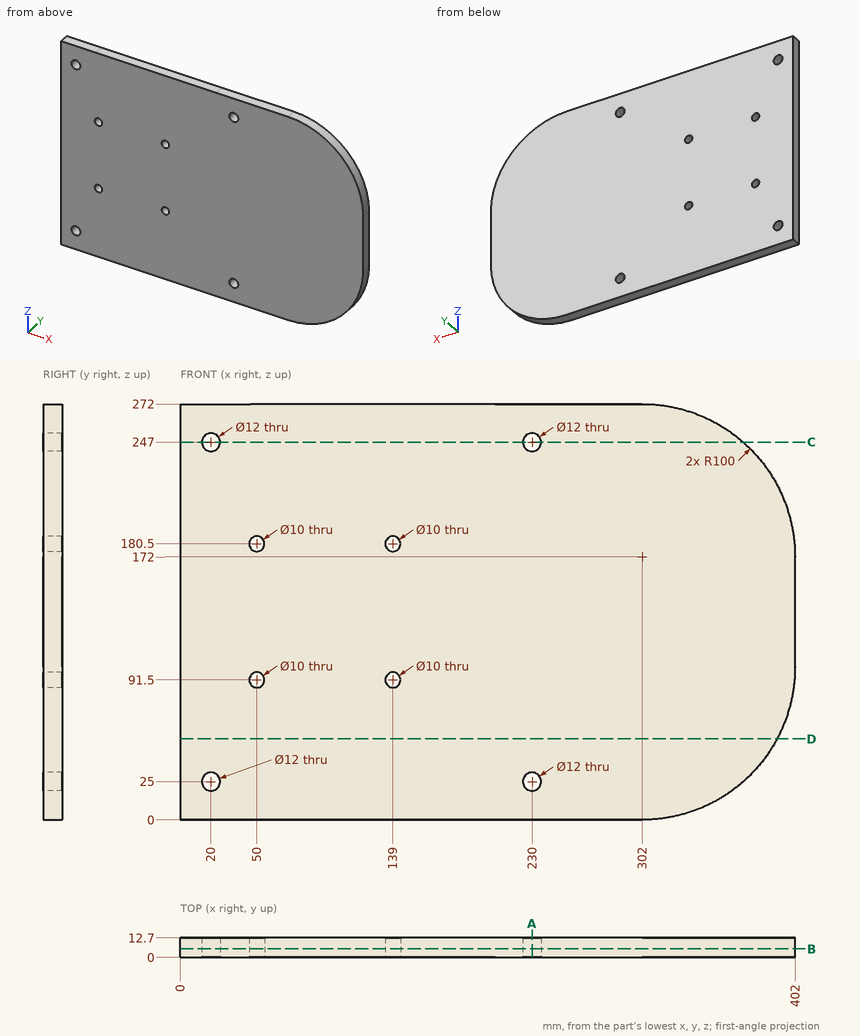
Geometry check sheet. Reference: drawing and pictorial views, mm from the part's lowest x, y, z. Round coordinates to 2 decimals unless told otherwise and drop trailing zeros. Order: outer loops, then holes, each group sorted by start corner. A loop starts at its lowest first (then second) coordinate and runs counter-clockwise, first axis right, second up. Notation, with made-up numbers: M 33,-28 L 44,-28 A30 cw 44,-2 Z; hole C -23,-32 d6. An arc over 180 degrees is marked long. Answer in a Markdown table with one row per item.
(1) Scan lines: probe 1 along Z at (x, y) = (50, 6.75); probe 2 along Z at (x, y) = (20, 9.75); probe 3 along X at (y, z) = (9.75, 180.5). Record each from-to range of solid material in increasing order. Write a range as from..to.
Responses:
| item | result |
|---|---|
| probe 1 | z = 0..86.5, 96.5..175.5, 185.5..272 |
| probe 2 | z = 0..19, 31..241, 253..272 |
| probe 3 | x = 0..45, 55..134, 144..401.64 |
(2) Sectioned sample at B-B, the plane y = 5.5. State how many separate pieces and enclosed holes the cut face has, and give its area (3 significant figures).
Responses:
| item | result |
|---|---|
| separate pieces | 1 |
| enclosed holes | 8 |
| area | 104,000 mm² |
(3) Go/stop test with flat-tipped pins: P1, Ø6, axis at y = 9, z = 63.5, coming from the +X side; P2, Ø14, axis at x = 20, z = 25, coming from the +Y side. Record where each tip stops, or that it passes through.
Responses:
| item | result |
|---|---|
| P1 | stops at x = 396.22 |
| P2 | stops at y = 12.7 |
(4) Sectioned sample at C-C, the plane z = 247. Record the cut outline in (x, y), and give its area (3 significant figures).
Responses:
| item | result |
|---|---|
| outline | M 0,0 L 14,0 L 14,12.7 L 0,12.7 Z; M 26,0 L 224,0 L 224,12.7 L 26,12.7 Z; M 236,0 L 368.14,0 L 368.14,12.7 L 236,12.7 Z |
| area | 4,370 mm² |
(5) Sectioned sample at A-A, the plane x = 230. Record the cut outline in (y, z).
Responses:
| item | result |
|---|---|
| outline | M 0,0 L 12.7,0 L 12.7,19 L 0,19 Z; M 0,31 L 12.7,31 L 12.7,241 L 0,241 Z; M 0,253 L 12.7,253 L 12.7,272 L 0,272 Z |
(6) Sectioned sample at D-D, the plane z = 53. Record the cut outline in (x, y).
Responses:
| item | result |
|---|---|
| outline | M 0,0 L 390.27,0 L 390.27,12.7 L 0,12.7 Z |
